Autodesk Inventor part; units mm, degrees
ref_plane "YZ Plane" through (0, 0, 0) normal (1, 0, 0) x (0, 1, 0)
ref_plane "XZ Plane" through (0, 0, 0) normal (0, 1, 0) x (-1, 0, 0)
ref_plane "XY Plane" through (0, 0, 0) normal (0, 0, 1) x (1, 0, 0)
sketch "Sketch1" plane through (0, 0, 0) normal (0, 1, 0) x (-1, 0, 0)
  line L0 (3.85, 4.1) -> (-3.85, 4.1)
  line L1 (-3.85, 4.1) -> (-3.85, -4.1)
  line L2 (-3.85, -4.1) -> (3.85, -4.1)
  line L3 (3.85, -4.1) -> (3.85, 4.1)
  line L4 (3.85, 4.1) -> (-3.85, -4.1) construction
  line L5 (-3.85, 4.1) -> (3.85, -4.1) construction
  circle A0 centre (0, 0) radius 2.8472
  dimension "d0" = 7.7
  dimension "d1" = 8.2
extrude "Extrusion1" add sketch "Sketch1" along normal blind 5
properties part number "00_Lens_Iphone_5s"
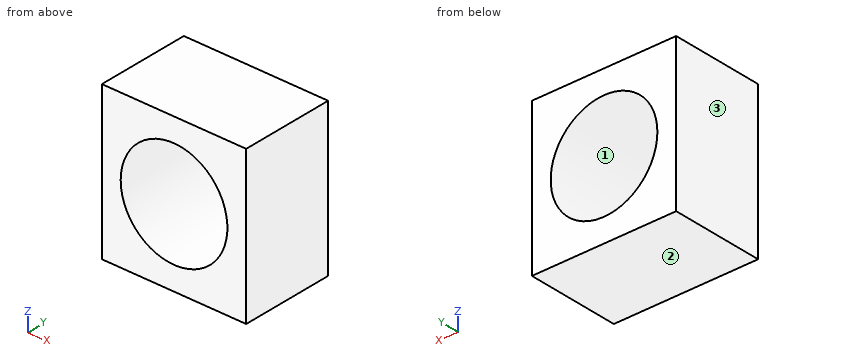
Can you work these out from the model? Positions are in its coordinate system, mm. Face numbers are marked on the shaded views. Give positions to 0.01 mm unless a question says otherwise; leave off trailing zeros. Order: outer loops, then holes, each group sorted by start corner. A loop starts at its lowest first (then second) coordinate and runs counter-clockwise, first axis right, second up. Notation, with made-up numbers: M 84,-0.5 L 101,-0.5 A28 ccw 101,20.5 Z; hole C 24.25,-12.75 d3. An arc over 180 degrees is marked long. One line per item, written item: value.
Item 1: If we mould it in two halves opening along X, with no side actions, what happens to the marked faces 1, 2 and 3? For each: pulls with the +X half, pulls with the -X half, needs draft (parallel to the pull), parting line crosses it, or undercut.
Verdict:
face 1: undercut
face 2: needs draft
face 3: pulls with the -X half
Item 2: Please list where these lines run through material, in increasing order: line 1 (Z direction, x = 0, y = 1); line 2 (X direction, y = 3.5, z = 1.25); line 3 (X direction, y = 3.35, z = 1.5).
Verdict:
line 1: -4.1 to -2.85, 2.85 to 4.1
line 2: -3.85 to -2.56, 2.56 to 3.85
line 3: -3.85 to -2.42, 2.42 to 3.85
Item 3: If we section it at A-A on z = 0: Write out the boundary of the cut face in (x, y).
Verdict:
outline: M -3.85,0 L -2.85,0 L -2.85,5 L -3.85,5 Z; M 2.85,0 L 3.85,0 L 3.85,5 L 2.85,5 Z
Item 4: If we section it at B-B on x = 2.5: Write out the boundary of the cut face in (y, z), and give its area (3 significant figures).
Verdict:
outline: M 0,-4.1 L 5,-4.1 L 5,-1.36 L 0,-1.36 Z; M 0,1.36 L 5,1.36 L 5,4.1 L 0,4.1 Z
area: 27.4 mm2
Item 5: If we section it at C-C on y = 4.7: Write out the boundary of the cut face in (x, z).
Verdict:
outline: M -3.85,-4.1 L 3.85,-4.1 L 3.85,4.1 L -3.85,4.1 Z; hole C 0,0 d5.69
